from build123d import *

# Parameters (mm, degrees)
SKETCH_1_W               = 20.2
SKETCH_1_H               = 20.2
EXTRUDE_1_DEPTH          = 1.63
FILLET_1_R               = 1
CUT_EXTRUDE_1_DEPTH      = 5
CUT_EXTRUDE_1_DEPTH_BACK = 15.376261684
SKETCH_2_R               = 1
EXTRUDE_2_DEPTH          = 2.5
EXTRUDE_3_DEPTH          = 2.6
SKETCH_6_W               = 7.6
SKETCH_6_H               = 0.5
EXTRUDE_6_DEPTH          = 6
SKETCH_7_W               = 7.6
SKETCH_7_H               = 6
EXTRUDE_7_DEPTH          = 0.4
SKETCH_8_W               = 7.6
SKETCH_8_H               = 6
CUT_EXTRUDE_2_DEPTH      = 0.4
EXTRUDE_8_DEPTH          = 1.4
SKETCH_10_W              = 6.8
SKETCH_10_H              = 1.6
CUT_EXTRUDE_3_DEPTH      = 1.5


with BuildPart() as part:
    # 草图1 → 凸台-拉伸1 (new body)
    with BuildSketch(Plane.XY):
        Rectangle(SKETCH_1_W, SKETCH_1_H)
    extrude(amount=EXTRUDE_1_DEPTH)

    # 圆角1
    fillet_1_edges = [part.edges().sort_by_distance(p)[0] for p in [
        (10.1, -10.1, 0.815),
        (-10.1, -10.1, 0.815),
        (-10.1, 10.1, 0.815),
        (10.1, 10.1, 0.815),
    ]]
    fillet(fillet_1_edges, radius=FILLET_1_R)

    # 草图2 → 切除-拉伸1 (cut, two sides: drawn at the far end of the back side and taken through both)
    with BuildSketch(Plane.XY.offset(1.63).offset(-CUT_EXTRUDE_1_DEPTH_BACK)):
        with Locations((-7.5, 7.5)):
            Circle(SKETCH_2_R)
        with Locations((7.5, 7.5)):
            Circle(SKETCH_2_R)
        with Locations((7.5, -7.5)):
            Circle(SKETCH_2_R)
        with Locations((-7.5, -7.5)):
            Circle(SKETCH_2_R)
    extrude(amount=CUT_EXTRUDE_1_DEPTH + CUT_EXTRUDE_1_DEPTH_BACK, mode=Mode.SUBTRACT)

    # 草图3 → 凸台-拉伸2 (add)
    with BuildSketch(Plane.XY.offset(1.63)):
        Polygon((0, 6.4), (3.8, 6.4), (3.8, 11.1), (-3.8, 11.1), (-3.8, 6.4), align=None)
    extrude(amount=EXTRUDE_2_DEPTH)

    # 草图4 → 凸台-拉伸3 (add)
    with BuildSketch(Plane.XY.offset(1.63)):
        Polygon((0, -8.1), (-2.25, -8.1), (-2.25, -0.6), (2.25, -0.6), (2.25, -8.1), align=None)
    extrude(amount=EXTRUDE_3_DEPTH)

    # 草图6 → 凸台-拉伸6 (add)
    with BuildSketch(Plane(origin=(0, 11.1, 0), x_dir=(1, 0, 0), z_dir=(0, 1, 0))):
        with Locations((0, -3.78)):
            Rectangle(SKETCH_6_W, SKETCH_6_H)
    extrude(amount=EXTRUDE_6_DEPTH)

    # 草图7 → 凸台-拉伸7 (add)
    with BuildSketch(Plane(origin=(0, 0, 3.53), x_dir=(-1, 0, 0), z_dir=(0, 0, -1))):
        with Locations((0, 14.1)):
            Rectangle(SKETCH_7_W, SKETCH_7_H)
    extrude(amount=EXTRUDE_7_DEPTH)

    # 草图8 → 切除-拉伸2 (cut)
    with BuildSketch(Plane.XY.offset(4.03)):
        with Locations((0, 14.1)):
            Rectangle(SKETCH_8_W, SKETCH_8_H)
    extrude(amount=-CUT_EXTRUDE_2_DEPTH, mode=Mode.SUBTRACT)

    # 草图9 → 凸台-拉伸8 (add)
    with BuildSketch(Plane(origin=(0, 0, 0), x_dir=(-1, 0, 0), z_dir=(0, 0, -1))):
        Polygon((-3.4, 6.1), (0, 6.1), (3.4, 6.1), (3.4, 7.7), (-3.4, 7.7), align=None)
    extrude(amount=EXTRUDE_8_DEPTH)

    # 草图10 → 切除-拉伸3 (cut)
    with BuildSketch(Plane(origin=(6.414908285, 4.302749918, 0), x_dir=(1, 0, 0), z_dir=(0, 0, 1))):
        with Locations((-6.414908285, 2.597250082)):
            Rectangle(SKETCH_10_W, SKETCH_10_H)
    extrude(amount=-CUT_EXTRUDE_3_DEPTH, mode=Mode.SUBTRACT)


solid = part.part
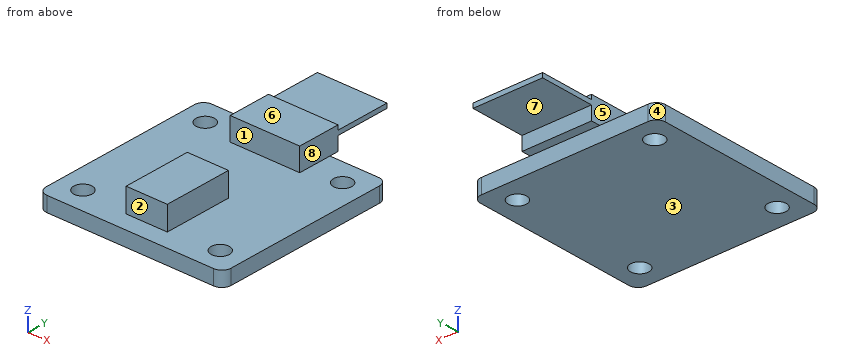
Can you work these out from the model? Positions are in its coordinate system, mm. Face numbers are marked on the shaded views. A direction names the side the tool comes from. Coordinates: 2 decimals unless noted, no trailing zeros. Write each loop counter-clockwise with the first axis right and the second up, starting at its lowest first coordinate (ties: lowest second). Pieces come first, ordered by that corner, then holes. Notation, with made-up numbers: (24.25, 84.5) - (35.25, 84.5) arc R18 ccw to (35.25, 107.5) - close; hole circle Ø9 at (40, 44.5). An arc over 180 degrees is marked (long way). Return JSON: item names as keys, results as strings. Group by question number.
Item 1: If we section it at B-B (x = -7.5): Write out the boundary of the cut face in (y, z), then the cut area to 3 significant figures.
Item 2: If we section it at C-C (z = 0.3): Write out the boundary of the cut face in (x, y).
Item 3: Please list where these lines run through material, in increasing order: probe 1 along Y at (x, z) = (7.5, 0.8); probe 2 along Y at (x, z) = (-0.75, 3.3).
Item 4: I'm going to push flat-ended pins straight in: pin 1 Ø2 at (x, z) = (-1, 1.5) entering from +Y; pin 2 Ø2 at (y, z) = (-6, 3.5) entering from -X; pin 3 Ø2 at (y, z) = (13.5, 2.5) entering from -X. Where does each tip first touch, or does it pass through?
Item 5: If we section it at A-A (z = 1.95): Write out the boundary of the cut face in (x, y), then the cut area to 3 significant figures.
Item 6: If we section it at D-D (y = -7.5): Write out the boundary of the cut face in (x, z), then the cut area to 3 significant figures.
Item 7: We'd pull the mould along Y, two halves only. Please class the marked faces 1, 2, 3 and 4: pulls with the +Y half, pulls with the -Y half, needs draft (parallel to the pull), parting line crosses it, or undercut.
Item 8: Which directions (+Z, -Z, +X, -X, +Y, -Y) give clear straight access to the entire face, cutting with the end or side of a thin tool? Please do the marked faces 5, 6, 7 and 8.
Return value:
{
 "1": {"outline": "(-10.1, 0) - (-8.5, 0) - (-8.5, 1.63) - (-10.1, 1.63) - close; (-6.5, 0) - (6.5, 0) - (6.5, 1.63) - (-6.5, 1.63) - close; (8.5, 0) - (10.1, 0) - (10.1, 1.63) - (8.5, 1.63) - close", "area": "26.4 mm^2"},
 "2": {"outline": "(-10.1, -9.1) arc R1 ccw to (-9.1, -10.1) - (9.1, -10.1) arc R1 ccw to (10.1, -9.1) - (10.1, 9.1) arc R1 ccw to (9.1, 10.1) - (-9.1, 10.1) arc R1 ccw to (-10.1, 9.1) - close; hole circle Ø2 at (-7.5, -7.5); hole circle Ø2 at (-7.5, 7.5); hole circle Ø2 at (7.5, -7.5); hole circle Ø2 at (7.5, 7.5)"},
 "3": {"probe 1": "y = -10.1 to -8.5, -6.5 to 6.5, 8.5 to 10.1", "probe 2": "y = -8.1 to -0.6, 6.4 to 17.1"},
 "4": {"pin 1": "stops at y = 11.1", "pin 2": "stops at x = -2.25", "pin 3": "stops at x = -3.8"},
 "5": {"outline": "(-3.8, 6.4) - (3.8, 6.4) - (3.8, 11.1) - (-3.8, 11.1) - close; (-2.25, -8.1) - (2.25, -8.1) - (2.25, -0.6) - (-2.25, -0.6) - close", "area": "69.5 mm^2"},
 "6": {"outline": "(-10.1, 0) - (-8.5, 0) - (-8.5, 1.63) - (-10.1, 1.63) - close; (-6.5, 0) - (6.5, 0) - (6.5, 1.63) - (2.25, 1.63) - (2.25, 4.23) - (-2.25, 4.23) - (-2.25, 1.63) - (-6.5, 1.63) - close; (8.5, 0) - (10.1, 0) - (10.1, 1.63) - (8.5, 1.63) - close", "area": "38.1 mm^2"},
 "7": {"face 1": "undercut", "face 2": "pulls with the -Y half", "face 3": "needs draft", "face 4": "pulls with the +Y half"},
 "8": {"face 5": "+Z, -X, +Y, -Y", "face 6": "+Z, +X, -X, +Y", "face 7": "-Z, +X, -X, +Y", "face 8": "+Z, +X, +Y, -Y"}
}
